from build123d import *

# Parameters (mm, degrees)
BOSS_EXTRUDE3_DEPTH = 30
SKETCH8_W           = 137
SKETCH8_H           = 101
BOSS_EXTRUDE5_DEPTH = 10
SKETCH9_W           = 57.5
SKETCH9_H           = 101
BOSS_EXTRUDE6_DEPTH = 8.5
SKETCH10_W          = 57.5
SKETCH10_H          = 101
SKETCH10_W_2        = 58
BOSS_EXTRUDE7_DEPTH = 8.5
SKETCH13_R          = 2.5
CUT_EXTRUDE1_DEPTH  = 8
SKETCH14_R          = 2.5
CUT_EXTRUDE2_DEPTH  = 8
SKETCH15_R          = 2.5
CUT_EXTRUDE3_DEPTH  = 8
SKETCH16_R          = 2.5
CUT_EXTRUDE4_DEPTH  = 8


with BuildPart() as part:
    # Sketch5 → Boss-Extrude3 (new body)
    with BuildSketch(Plane(origin=(0, 0, 0), x_dir=(1, 0, 0), z_dir=(0, 1, 0))):
        Polygon((100, 199), (100, 300), (0, 300), (0, 0), (100, 0), (100, 101), (237, 101), (237, 0), (337, 0), (337, 300), (237, 300), (237, 199), align=None)
    extrude(amount=BOSS_EXTRUDE3_DEPTH)

    # Sketch8 → Boss-Extrude5 (add)
    with BuildSketch(Plane(origin=(0, 30, 0), x_dir=(1, 0, 0), z_dir=(0, 1, 0))):
        with Locations((168.5, 249.5)):
            Rectangle(SKETCH8_W, SKETCH8_H)
        with Locations((168.5, 50.5)):
            Rectangle(SKETCH8_W, SKETCH8_H)
    extrude(amount=-BOSS_EXTRUDE5_DEPTH)

    # Sketch9 → Boss-Extrude6 (add)
    with BuildSketch(Plane(origin=(0, 20, 0), x_dir=(1, 0, 0), z_dir=(0, 1, 0))):
        with Locations((128.75, 50.5)):
            Rectangle(SKETCH9_W, SKETCH9_H)
        with Locations((208.25, 50.5)):
            Rectangle(SKETCH9_W, SKETCH9_H)
    extrude(amount=-BOSS_EXTRUDE6_DEPTH)

    # Sketch10 → Boss-Extrude7 (add)
    with BuildSketch(Plane(origin=(0, 20, 0), x_dir=(1, 0, 0), z_dir=(0, 1, 0))):
        with Locations((128.75, 249.5)):
            Rectangle(SKETCH10_W, SKETCH10_H)
        with Locations((208, 249.5)):
            Rectangle(SKETCH10_W_2, SKETCH10_H)
    extrude(amount=-BOSS_EXTRUDE7_DEPTH)

    # Sketch13 → Cut-Extrude1 (cut)
    with BuildSketch(Plane.XZ.offset(-11.5)):
        with Locations((147.5, -8.5)):
            Circle(SKETCH13_R)
        with Locations((147.5, -92.5)):
            Circle(SKETCH13_R)
    extrude(amount=-CUT_EXTRUDE1_DEPTH, mode=Mode.SUBTRACT)

    # Sketch14 → Cut-Extrude2 (cut)
    with BuildSketch(Plane.XZ.offset(-11.5)):
        with Locations((189.5, -8.5)):
            Circle(SKETCH14_R)
        with Locations((189.5, -92.5)):
            Circle(SKETCH14_R)
    extrude(amount=-CUT_EXTRUDE2_DEPTH, mode=Mode.SUBTRACT)

    # Sketch15 → Cut-Extrude3 (cut)
    with BuildSketch(Plane.XZ.offset(-11.5)):
        with Locations((147.5, -207.5)):
            Circle(SKETCH15_R)
        with Locations((147.5, -291.5)):
            Circle(SKETCH15_R)
    extrude(amount=-CUT_EXTRUDE3_DEPTH, mode=Mode.SUBTRACT)

    # Sketch16 → Cut-Extrude4 (cut)
    with BuildSketch(Plane.XZ.offset(-11.5)):
        with Locations((189.5, -207.5)):
            Circle(SKETCH16_R)
        with Locations((189.5, -291.5)):
            Circle(SKETCH16_R)
    extrude(amount=-CUT_EXTRUDE4_DEPTH, mode=Mode.SUBTRACT)


solid = part.part
Could you check a few things on this model? Use its own coordinates, in mm. A direction names the side the tool comes from. Round coordinates to 2 decimals unless told otherwise and drop trailing zeros. Write each loop counter-clockwise with the first axis right and the second up, starting at its lowest first coordinate (ties: lowest second). Pieces come first, ordered by that corner, then holes. Notation, with made-up numbers: (29.25, 38.5) - (85.25, 38.5) arc R20 cw to (85.25, 59.5) - close; hole circle Ø2 at (61, 10.5). An arc over 180 degrees is marked (long way). Put each result on its own line as item: value. Start each with the question number.
(1) Will these pins go through, and if not, where does the flat tip stop? pin 1 (8 mm diameter, centred on x = 195, z = -234, fed in from -Y); pin 2 (11 mm diameter, centred on x = 171, z = -261, fed in from -Y); pin 3 (6 mm diameter, centred on x = 162, y = 14, fed in from -Z).
(2) I want a section at A-A, the plane z = -237. Please give me the cut outline in (x, y).
(3) For faces 4 (the flat face through (100, 6, -50)), 5 (the flat face through (237, 6, -250)), 6 (the flat face through (166, 0, -152)), which set-ups out of +Z, -Z, +X, -X, +Y, -Y let a thin tool reach every point of the face, with its end or its side?
(4) I want a section at B-B, the plane z = -25. Please give me the cut outline in (x, y), plus the area to 3 significant figures.
(5) I need wall thicknesses on probe 1 along Z at (x, y) = (189.5, 15.5); probe 2 along X at (y, z) = (14.75, -291.5); probe 3 along X at (y, z) = (6.5, -234.5). Which ranges of each line are inside material? Lowest first, please.
(6) Thinking about a two-plate mould opening in X: for faces 1 (the flat face through (0, 15, -152)), 2 (the flat face through (166, 22, -300)), 3 (the flat face through (179.5, 16, -50)), which applies, released by +X, released by -X, zero draft, split by the parting line, or undercut?
Here are the results:
1. pin 1: stops at y = 11.5
1. pin 2: stops at y = 20
1. pin 3: stops at z = -199
2. outline: (0, 0) - (100, 0) - (100, 11.5) - (157.5, 11.5) - (157.5, 20) - (179, 20) - (179, 11.5) - (237, 11.5) - (237, 0) - (337, 0) - (337, 30) - (0, 30) - close
3. face 4: +Z, -Y
3. face 5: -Z, -Y
3. face 6: +Z, -Z, +X, -X, -Y
4. outline: (0, 0) - (100, 0) - (100, 11.5) - (157.5, 11.5) - (157.5, 20) - (179.5, 20) - (179.5, 11.5) - (237, 11.5) - (237, 0) - (337, 0) - (337, 30) - (0, 30) - close
4. area: 8,350 mm^2
5. probe 1: z = -300 to -294, -289 to -210, -205 to -95, -90 to -11, -6 to 0
5. probe 2: x = 0 to 145, 150 to 157.5, 179 to 187, 192 to 337
5. probe 3: x = 0 to 100, 237 to 337
6. face 1: released by -X
6. face 2: zero draft
6. face 3: undercut
